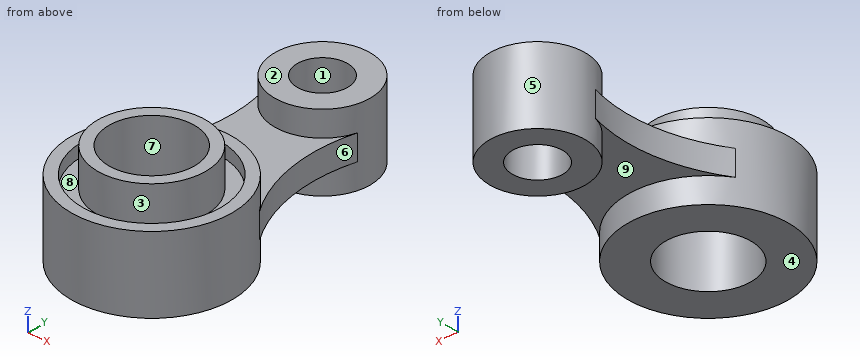
```python
from build123d import *

# Parameters (mm, degrees)
SKETCH2_R                = 32
SKETCH2_R_2              = 27.5
BOSS_EXTRUDE1_DEPTH      = 30
BOSS_EXTRUDE2_DEPTH      = 5
BOSS_EXTRUDE2_DEPTH_BACK = 5
BOSS_EXTRUDE3_DEPTH      = 15
BOSS_EXTRUDE3_DEPTH_BACK = 15
SKETCH4_R                = 19
SKETCH4_R_2              = 10
BOSS_EXTRUDE4_DEPTH      = 10
BOSS_EXTRUDE4_DEPTH_BACK = 15
SKETCH5_R                = 27.5
SKETCH6_R                = 21.5
BOSS_EXTRUDE5_DEPTH      = 15
SKETCH7_R                = 17
CUT_EXTRUDE1_DEPTH       = 40


with BuildPart() as part:
    # Sketch2 → Boss-Extrude1 (new body)
    with BuildSketch(Plane.XY):
        Circle(SKETCH2_R)
        Circle(SKETCH2_R_2, mode=Mode.SUBTRACT)
    extrude(amount=BOSS_EXTRUDE1_DEPTH)

    # Sketch3 → Boss-Extrude2 (add, two sides: drawn at the far end of the back side and taken through both)
    with BuildSketch(Plane.XY.offset(15).offset(-BOSS_EXTRUDE2_DEPTH_BACK)):
        with BuildLine():
            ThreePointArc((-18.321243986, 69.966907631), (0, 56), (18.321243986, 69.966907631))
            ThreePointArc((18.321243986, 69.966907631), (16.836772686, 42.914041255), (26.678302647, 17.671111111))
            ThreePointArc((26.678302647, 17.671111111), (0, 32), (-26.678302647, 17.671111111))
            ThreePointArc((-26.678302647, 17.671111111), (-16.836772686, 42.914041255), (-18.321243986, 69.966907631))
        make_face()
    extrude(amount=BOSS_EXTRUDE2_DEPTH + BOSS_EXTRUDE2_DEPTH_BACK)

    # Sketch4 → Boss-Extrude3 (add, two sides: drawn at the far end of the back side and taken through both)
    with BuildSketch(Plane.XY.offset(15).offset(-BOSS_EXTRUDE3_DEPTH_BACK)):
        with Locations((0, 75)):
            Circle(SKETCH4_R)
        with Locations((0, 75)):
            Circle(SKETCH4_R_2, mode=Mode.SUBTRACT)
    extrude(amount=BOSS_EXTRUDE3_DEPTH + BOSS_EXTRUDE3_DEPTH_BACK)

    # Sketch5 → Boss-Extrude4 (add, two sides: drawn at the far end of the back side and taken through both)
    with BuildSketch(Plane.XY.offset(15).offset(-BOSS_EXTRUDE4_DEPTH_BACK)):
        Circle(SKETCH5_R)
    extrude(amount=BOSS_EXTRUDE4_DEPTH + BOSS_EXTRUDE4_DEPTH_BACK)

    # Sketch6 → Boss-Extrude5 (add)
    with BuildSketch(Plane.XY.offset(25)):
        Circle(SKETCH6_R)
    extrude(amount=BOSS_EXTRUDE5_DEPTH)

    # Sketch7 → Cut-Extrude1 (cut)
    with BuildSketch(Plane.XY.offset(40)):
        Circle(SKETCH7_R)
    extrude(amount=-CUT_EXTRUDE1_DEPTH, mode=Mode.SUBTRACT)


solid = part.part
```
The listing builds one solid part. Answer for the finished solid, in the listing's coordinates (mm). Face numbers are marked on the shaded views. A direction names the side the tool comes from. Give positions to 0.01 mm unless a question says otherwise; leave off trailing zeros. Order: outer loops, then holes, each group sorted by start corner. A loop starts at its lowest first (then second) coordinate and runs counter-clockwise, first axis right, second up.
1) For the marked faces 1, 2, 3, 4 and 5, determine the directions among +Z, -Z, +X, -X, +Y, -Y from which every point of the face is accessible in a straight line to the end or side of a thin tool.
Reported:
face 1: +Z, -Z
face 2: +Z, +X, -X, +Y
face 3: +Z
face 4: -Z, +X, -X, +Y, -Y
face 5: none
2) Find section D-D on x = -13.5. Write down the section's boundary in (y, z).
Reported:
outline: (-29.01, 0) - (-10.33, 0) - (-10.33, 40) - (-16.73, 40) - (-16.73, 25) - (-23.96, 25) - (-23.96, 30) - (-29.01, 30) - close; (10.33, 0) - (29.01, 0) - (29.01, 10) - (61.63, 10) - (61.63, 0) - (88.37, 0) - (88.37, 30) - (61.63, 30) - (61.63, 20) - (29.01, 20) - (29.01, 30) - (23.96, 30) - (23.96, 25) - (16.73, 25) - (16.73, 40) - (10.33, 40) - close
3) Find section A-A on x = 0. Write down the section's boundary in (y, z), then the cut area to 3 significant figures.
Reported:
outline: (-32, 0) - (-17, 0) - (-17, 40) - (-21.5, 40) - (-21.5, 25) - (-27.5, 25) - (-27.5, 30) - (-32, 30) - close; (17, 0) - (32, 0) - (32, 10) - (56, 10) - (56, 0) - (65, 0) - (65, 30) - (56, 30) - (56, 20) - (32, 20) - (32, 30) - (27.5, 30) - (27.5, 25) - (21.5, 25) - (21.5, 40) - (17, 40) - close; (85, 0) - (94, 0) - (94, 30) - (85, 30) - close
area: 1,710 mm2
4) Given P1, Ø6, axis at x = -19, y = 55.5, coming from the +Z side; P2, Ø6, axis at x = 9, z = 32, coming from the -Y side; P3, Ø12, axis at y = 64, z = 11, coming from the +X side; P4, Ø12, axis at x = 10, y = -2, coming from the -Z side, each flat-ended and moving along its own axis, determine where each tip first touches the part or whether it passes through.
Reported:
P1: stops at z = 20
P2: stops at y = -31.28
P3: stops at x = 18.33
P4: passes through
5) Find section C-C on z = 26.5. Write down the section's boundary in (x, y).
Reported:
outline: circle Ø64 at (0, 0); circle Ø43 at (0, 0); circle Ø38 at (0, 75); hole circle Ø55 at (0, 0); hole circle Ø34 at (0, 0); hole circle Ø20 at (0, 75)
6) Determine the mould class of the marked faces 6, 7, 8 and 9 for opening direction X: pulls with the +X half, pulls with the -X half, needs draft (parallel to the pull), parting line crosses it, or undercut.
Reported:
face 6: pulls with the +X half
face 7: undercut
face 8: undercut
face 9: needs draft
7) Consider line 1 along Y through (x, z) = (0, 27); line 2 along Y through (x, z) = (0, 6); line 3 along Y through (x, z) = (11, 28). Determine where each line is inside the solid, lowest interval first.
Reported:
line 1: y = -32 to -27.5, -21.5 to -17, 17 to 21.5, 27.5 to 32, 56 to 65, 85 to 94
line 2: y = -32 to -17, 17 to 32, 56 to 65, 85 to 94
line 3: y = -30.05 to -25.2, -18.47 to -12.96, 12.96 to 18.47, 25.2 to 30.05, 59.51 to 90.49
8) Find section B-B on y = 75. Write down the section's boundary in (x, z).
Reported:
outline: (-19, 0) - (-10, 0) - (-10, 30) - (-19, 30) - close; (10, 0) - (19, 0) - (19, 30) - (10, 30) - close
